```python
from build123d import *

# Parameters (mm, degrees)
CUT_EXTRUDE1_DEPTH = 0.6
SKETCH4_R          = 0.9375
CUT_EXTRUDE2_DEPTH = 0.8
CUT_EXTRUDE2_DRAFT = -45


with BuildPart() as part:
    # Sketch2 → Revolve1 (revolve)
    with BuildSketch(Plane(origin=(0, 0, 0), x_dir=(0, 0, -1), z_dir=(1, 0, 0)), mode=Mode.PRIVATE) as revolve1_sk:
        with BuildLine():
            Line((-5.8, 0), (-5.8, 1.42))
            Line((-5.8, 1.42), (-5.72, 1.5))
            Line((-5.72, 1.5), (-4.28, 1.5))
            Line((-4.28, 1.5), (-4.2, 1.42))
            Line((-4.2, 1.42), (-4.2, 1))
            ThreePointArc((-4.2, 1), (-4.141421356, 0.858578644), (-4, 0.8))
            Line((-4, 0.8), (5.572668332, 0.8))
            Line((5.572668332, 0.8), (5.8, 0.572668332))
            Line((5.8, 0.572668332), (5.8, 0))
            Line((5.8, 0), (-5.8, 0))
        make_face()
    revolve(revolve1_sk.sketch.rotate(Axis((0, 0, -5.8), (0, 0, 1)), 90), axis=Axis((0, 0, -5.8), (0, 0, 1)))

    # Sketch3 → Cut-Extrude1 (cut)
    with BuildSketch(Plane.XY.offset(5.8)):
        Polygon((0.75, -0.433012702), (0.75, 0.433012702), (0, 0.866025404), (-0.75, 0.433012702), (-0.75, -0.433012702), (0, -0.866025404), align=None)
    extrude(amount=-CUT_EXTRUDE1_DEPTH, mode=Mode.SUBTRACT)


with BuildPart() as cut_extrude2_tool:
    # Sketch4 → Cut-Extrude2 (with draft: the straight prism first)
    with BuildSketch(Plane.XY.offset(5.8)):
        Circle(SKETCH4_R)
    extrude(amount=-CUT_EXTRUDE2_DEPTH)
    # Cut-Extrude2: the draft: its side faces are tilted about the plane it starts from
    cut_extrude2_sides = [cut_extrude2_tool.faces().sort_by_distance(p)[0] for p in [
        (-0.9375, 0, 5.4),
    ]]
    draft(cut_extrude2_sides, Plane.XY.offset(5.8), CUT_EXTRUDE2_DRAFT)


with BuildPart() as part_1:
    add(part.part)

    # Cut-Extrude2: cut by cut_extrude2_tool
    add(cut_extrude2_tool.part, mode=Mode.SUBTRACT)


solid = part_1.part
```
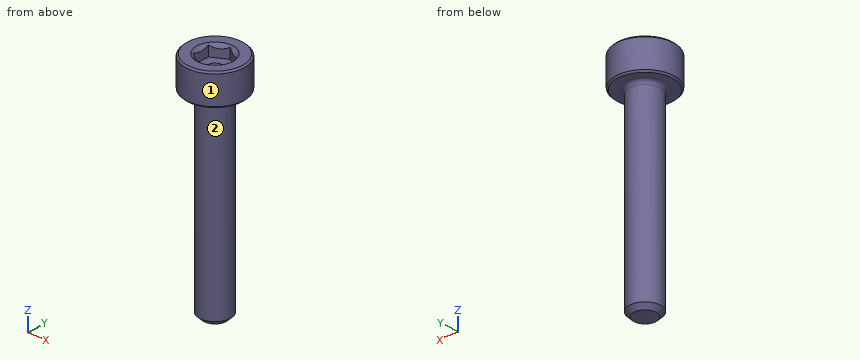
Could you check a few things on this model? Use its own coordinates, in mm. Face numbers are marked on the shaded views. A direction names the side the tool comes from. Round coordinates to 2 decimals unless told otherwise and drop trailing zeros. Write each loop counter-clockwise with the first axis right and the second up, starting at its lowest first coordinate (ties: lowest second). Pieces come first, ordered by that corner, then holes.
(1) If I drill on probe 1 along X at (y, z) = (-0.05, -4.5); probe 2 along Z at (x, y) = (-1.15, 0.05); probe 3 along Z at (x, y) = (-0.2, 0.35), over which ranges is the centre line in solid material (lowest first)?
Findings below:
probe 1: x = -0.8 to 0.8
probe 2: z = 4.2 to 5.8
probe 3: z = -5.8 to 5.2
(2) Suppose I cut it at B-B on z = -4.25. Write out the boundary of the cut face in (x, y), and give its area (3 significant figures).
Findings below:
outline: circle Ø1.6 at (0, 0)
area: 2.01 mm2
(3) Which directions (+Z, -Z, +X, -X, +Y, -Y) give clear straight access to the entire face, cutting with the end or side of a thin tool? Please do the marked faces 1 and 2.
Findings below:
face 1: +Z, -Z
face 2: -Z
(4) Suppose I cut it at A-A on y = 0. Write out the boundary of the cut face in (x, z).
Findings below:
outline: (-1.5, 4.28) - (-1.42, 4.2) - (-1, 4.2) arc R0.2 cw to (-0.8, 4) - (-0.8, -5.57) - (-0.57, -5.8) - (0.57, -5.8) - (0.8, -5.57) - (0.8, 4) arc R0.2 cw to (1, 4.2) - (1.42, 4.2) - (1.5, 4.28) - (1.5, 5.72) - (1.42, 5.8) - (0.94, 5.8) - (0.75, 5.61) - (0.75, 5.2) - (0.34, 5.2) - (0.14, 5) - (-0.14, 5) - (-0.34, 5.2) - (-0.75, 5.2) - (-0.75, 5.61) - (-0.94, 5.8) - (-1.42, 5.8) - (-1.5, 5.72) - close
(5) For pin 1 (1.4 mm diameter, centred on x = 0.5, y = 0.5, fed in from -Z); pin 2 (1 mm diameter, centred on y = -0.5, z = -1.5, fed in from +X), each with a flat end and sliding along its axis, tell me the tip position at first contact or that it passes through.
Findings below:
pin 1: stops at z = -5.8
pin 2: stops at x = 0.8
